from build123d import *

# Parameters (mm, degrees)
F0_W     = 310
F0_H     = 100
F1_DEPTH = 10
F3_DEPTH = 5


with BuildPart() as f1:
    # F0 (on Right) → F1 (new body)
    with BuildSketch(Plane.YZ):
        with Locations((0, 50)):
            Rectangle(F0_W, F0_H)
    extrude(amount=F1_DEPTH)

    # F2 (on face) → F3 (cut)
    with BuildSketch(Plane.YZ.offset(10)):
        Polygon((-125, 100), (-135, 100), (-135, 10), (0, 10), (135, 10), (135, 100), (125, 100), (125, 20), (0, 20), (-125, 20), align=None)
    extrude(amount=-F3_DEPTH, mode=Mode.SUBTRACT)


solid = f1.part
Could you check a few things on this model? Use its own coordinates, in mm. A direction names the side the tool comes from. Coordinates: 2 decimals unless noted, no trailing zeros. Loops run counter-clockwise (first coordinate to the right, second up) from the corner with the lowest first, then second, coordinate; pieces in that order, holes last. Notation, with made-up numbers: (89.5, 83) -> (142.5, 83) arc R22 cw to (142.5, 89) -> close; hole circle Ø4 at (69, -21.5). An arc over 180 degrees is marked (long way). Answer in a Markdown table with one row per item.
(1) Imagine slicing it at A-A (x = 8.25). List the corners of the cut face in (y, z) for me.
Results found:
| item | result |
|---|---|
| outline | (-155, 0) -> (155, 0) -> (155, 100) -> (135, 100) -> (135, 10) -> (-135, 10) -> (-135, 100) -> (-155, 100) -> close; (-125, 20) -> (125, 20) -> (125, 100) -> (-125, 100) -> close |
(2) For faces 4 (the face through (8, -125, 59)), 5 (the face through (5, -2, 0)), 6 (the face through (8, -2, 10)), which set-ups out of +Z, -Z, +X, -X, +Y, -Y let a thin tool reach every point of the face, with its end or its side?
Results found:
| item | result |
|---|---|
| face 4 | +Z, +X |
| face 5 | -Z, +X, -X, +Y, -Y |
| face 6 | +X |
(3) If I drill on probe 1 along Y at (x, z) = (6.5, 77.5); probe 2 along Z at (x, y) = (8.5, -59.5), over which ranges is the centre line in solid material (lowest first)?
Results found:
| item | result |
|---|---|
| probe 1 | y = -155 to -135, -125 to 125, 135 to 155 |
| probe 2 | z = 0 to 10, 20 to 100 |
(4) Imagine slicing it at D-D (z = 16.5). List the corners of the cut face in (x, y) for me, plus the area to 3 significant figures.
Results found:
| item | result |
|---|---|
| outline | (0, -155) -> (10, -155) -> (10, -135) -> (5, -135) -> (5, 135) -> (10, 135) -> (10, 155) -> (0, 155) -> close |
| area | 1,750 mm^2 |
(5) Imagine slicing it at B-B (z = 45.5). List the corners of the cut face in (x, y) for me.
Results found:
| item | result |
|---|---|
| outline | (0, -155) -> (10, -155) -> (10, -135) -> (5, -135) -> (5, -125) -> (10, -125) -> (10, 125) -> (5, 125) -> (5, 135) -> (10, 135) -> (10, 155) -> (0, 155) -> close |
(6) Thinking about a two-plate mould opening in Z: for faces 1 (the face through (8, 135, 54)), 2 (the face through (5, -1, 15)), 3 (the face through (5, -2, 100)), which applies, released by +Z, released by -Z, zero draft, split by the parting line, or undercut?
Results found:
| item | result |
|---|---|
| face 1 | zero draft |
| face 2 | undercut |
| face 3 | released by +Z |
(7) Imagine slicing it at C-C (y = 113). List the corners of the cut face in (x, z) for me.
Results found:
| item | result |
|---|---|
| outline | (0, 0) -> (10, 0) -> (10, 10) -> (5, 10) -> (5, 20) -> (10, 20) -> (10, 100) -> (0, 100) -> close |
(8) Will this pin go through, and if not, where does the flat tip stop? pin 1 Ø4 at (y, z) = (-88.5, 17) entering from +X.
Results found:
| item | result |
|---|---|
| pin 1 | stops at x = 5 |
